Answer from the drawing. Dimensions are ordinates in mm from the lowest x, y and z of the part. Round coordinates to 2 decimals unless told otherwise and drop trailing zeros. Write each loop counter-clockwise with the first axis right and the second up, starting at its lowest first coordinate (ties: lowest second). Pieces come first, ordered by that corner, then holes. Notation, with made-up numbers: (-25.5, -2.5) - (-21.5, -2.5) arc R32 ccw to (-21.5, 30.5) - close; hole circle Ø11 at (12, -26.5). An arc over 180 degrees is marked (long way). One line per item, written item: value. Start each with the question number.
(1) Flat-ended cylindrical pins translate along their axes: pin 1 Ø7 at (x, z) = (120.65, 31.75) entering from -Y; pin 2 Ø9 at (x, z) = (23.03, 76.2) entering from -Y; pin 3 Ø6 at (x, y) = (91.5, 52) entering from -Z; pin 4 Ø7 at (x, z) = (31.75, 120.65) entering from +Y. Find the tip coordinate at first contact, or state that the pin passes through.
(2) A cutting plane is placed at D-D, the plane z = 142. Determine the outline of the cut face in (x, y).
(3) Find the intervals of material crossed by L1, parallel to Z at x = 34, y = 71 (1 decimal); L2, parallel to Y at x = 105.5, z = 10; L3, parallel to Z at x = 76.2, y = 49.5 (3 decimals), in increasing order.
(4) A cutting plane is placed at B-B, the plane z = 120.65. Determine the outline of the cut face in (x, y), plus the area to 3 significant figures.
(5) The mould has two halves that part along Y. Classify the marked faces 1, 2, 3 and 4: +Y half, -Y half, draft (parallel to the pull), parting line (faces both ways), or undercut.
(6) A cutting plane is placed at C-C, the plane x = 130.5. State how many separate pieces and enclosed holes the cut face has, plus the area to 3 significant figures.
(7) A cutting plane is placed at A-A, the plane x = 87. Determine the outline of the cut face in (y, z).
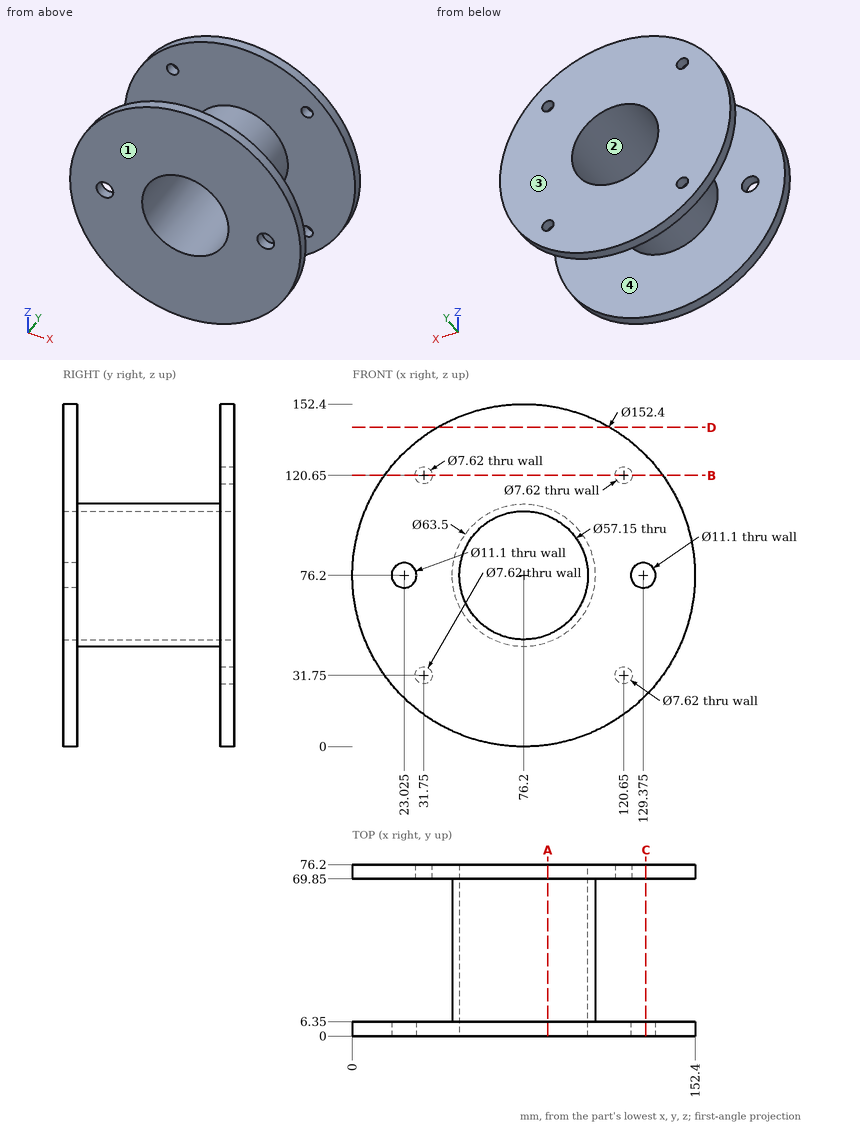
Here are the results:
1. pin 1: y = 0
1. pin 2: y = 69.85
1. pin 3: z = 46.93
1. pin 4: y = 6.35
2. outline: (37.77, 0) - (114.63, 0) - (114.63, 6.35) - (37.77, 6.35) - close; (37.77, 69.85) - (114.63, 69.85) - (114.63, 76.2) - (37.77, 76.2) - close
3. L1: 12.8 to 28.7, 34.8 to 117.6, 123.7 to 139.6
3. L2: 0 to 6.35, 69.85 to 76.2
3. L3: 44.45 to 47.625, 104.775 to 107.95
4. outline: (14.31, 0) - (138.09, 0) - (138.09, 6.35) - (14.31, 6.35) - close; (14.31, 69.85) - (27.94, 69.85) - (27.94, 76.2) - (14.31, 76.2) - close; (35.56, 69.85) - (116.84, 69.85) - (116.84, 76.2) - (35.56, 76.2) - close; (124.46, 69.85) - (138.09, 69.85) - (138.09, 76.2) - (124.46, 76.2) - close
4. area: 1,480 mm²
5. face 1: -Y half
5. face 2: draft
5. face 3: +Y half
5. face 4: undercut
6. separate pieces: 3
6. enclosed holes: 0
6. area: 1,290 mm²
7. outline: (0, 0.77) - (6.35, 0.77) - (6.35, 46.34) - (69.85, 46.34) - (69.85, 0.77) - (76.2, 0.77) - (76.2, 49.74) - (0, 49.74) - close; (0, 102.66) - (76.2, 102.66) - (76.2, 151.63) - (69.85, 151.63) - (69.85, 106.06) - (6.35, 106.06) - (6.35, 151.63) - (0, 151.63) - close
